Verification items for the finished model (mm, model axes). Face numbers are marked on the shaded views. Round coordinates to 2 decimals unless told otherwise and drop trailing zeros. Order: outer loops, then holes, each group sorted by start corner. A loop starts at its lowest first (then second) coordinate and runs counter-clockwise, first axis right, second up. Notation, with made-up numbers: (65.25, -16.5) -> (123.25, -16.5) arc R14 ccw to (123.25, -7.5) -> close; hole circle Ø2 at (4.5, -28.5). An arc over 180 degrees is marked (long way). Return JSON: item names as keys, results as strings. Group by question number.
Item 1: Sectioned sample at B-B on x = 0. Record the cut outline in (y, z).
Item 2: Depth check by flat-ended pin: pin 1 Ø2 at (y, z) = (17.5, 7.5) entering from -X; pin 2 Ø8 at (x, z) = (6.5, 18) entering from -Y; pin 3 Ø10 at (x, y) = (-31, 37.5) entering from +Z. Enter the tip coordinate at first touch or a pass-through.
Item 3: Sectioned sample at A-A on y = 0. Record the cut outline in (x, z), plus the area to 3 significant figures.
Item 4: Sectioned sample at D-D on z = 48. Record the cut outline in (x, y) (3 decimals), plus the area to 3 significant figures.
Item 5: Sectioned sample at C-C on z = 33. Give the number of separate pieces and of enclosed holes in the cut face, plus the area to 3 significant figures.
Item 6: Scan lines: probe 1 along Y at (x, z) = (0, 23.5); probe 2 along Y at (x, z) = (22.5, 36.5); probe 3 along X at (y, z) = (-5, 31). Record each from-to range of solid material in increasing order. Write a range as from..to.
Item 7: Draft check along X on the marked faces 1, 2 and 3. Enter one of: pulls with the +X half, pulls with the -X half, needs draft (parallel to the pull), parting line crosses it, or undercut.
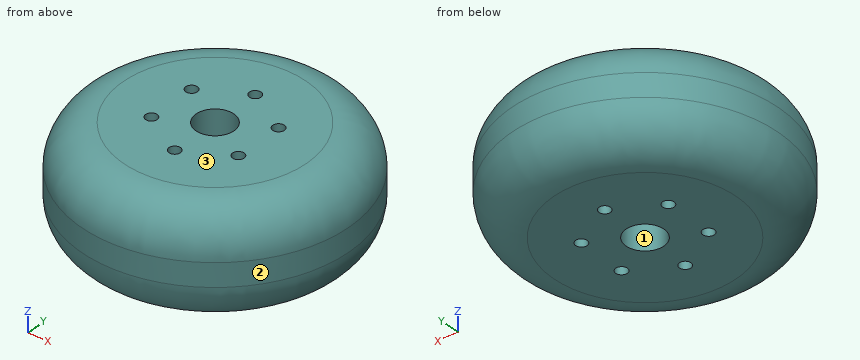
```python
from build123d import *

# Parameters (mm, degrees)
SKETCH1_R            = 63.5
SKETCH1_R_2          = 9
BOSS_EXTRUDE1_DEPTH  = 51
FILLET1_R            = 20
M5_CLEARANCE_HOLE1_D = 5.5


with BuildPart() as part:
    # Sketch1 → Boss-Extrude1 (new body)
    with BuildSketch(Plane.XY):
        Circle(SKETCH1_R)
        Circle(SKETCH1_R_2, mode=Mode.SUBTRACT)
    extrude(amount=BOSS_EXTRUDE1_DEPTH)

    # Fillet1
    fillet1_edges = [part.edges().sort_by_distance(p)[0] for p in [
        (-63.5, 0, 0),
        (-63.5, 0, 51),
    ]]
    fillet(fillet1_edges, radius=FILLET1_R)

    # M5 Clearance Hole1 (through all)
    with Locations(Plane.XY.offset(51)):
        with Locations((0, 23.75), (20.56810334, 11.875), (20.56810334, -11.875), (0, -23.75), (-20.56810334, -11.875), (-20.56810334, 11.875)):
            Hole(M5_CLEARANCE_HOLE1_D / 2)


solid = part.part
```
Recorded:
{
 "1": {"outline": "(-63.5, 20) arc R20 ccw to (-43.5, 0) -> (-26.5, 0) -> (-26.5, 51) -> (-43.5, 51) arc R20 ccw to (-63.5, 31) -> close; (-21, 0) -> (-9, 0) -> (-9, 51) -> (-21, 51) -> close; (9, 0) -> (21, 0) -> (21, 51) -> (9, 51) -> close; (26.5, 0) -> (43.5, 0) arc R20 ccw to (63.5, 20) -> (63.5, 31) arc R20 ccw to (43.5, 51) -> (26.5, 51) -> close"},
 "2": {"pin 1": "x = -57.31", "pin 2": "y = -63.43", "pin 3": "z = 51"},
 "3": {"outline": "(-63.5, 20) arc R20 ccw to (-43.5, 0) -> (-9, 0) -> (-9, 51) -> (-43.5, 51) arc R20 ccw to (-63.5, 31) -> close; (9, 0) -> (43.5, 0) arc R20 ccw to (63.5, 20) -> (63.5, 31) arc R20 ccw to (43.5, 51) -> (9, 51) -> close", "area": "5,220 mm²"},
 "4": {"outline": "circle Ø108.071 at (0, 0); hole circle Ø5.5 at (-20.568, -11.875); hole circle Ø5.5 at (-20.568, 11.875); hole circle Ø18 at (0, 0); hole circle Ø5.5 at (0, -23.75); hole circle Ø5.5 at (0, 23.75); hole circle Ø5.5 at (20.568, -11.875); hole circle Ø5.5 at (20.568, 11.875)", "area": "8,780 mm²"},
 "5": {"separate pieces": "1", "enclosed holes": "7", "area": "12,200 mm²"},
 "6": {"probe 1": "-63.5..-26.5, -21..-9, 9..21, 26.5..63.5", "probe 2": "-58.55..-13.83, -9.92..9.92, 13.83..58.55", "probe 3": "-63.3..-7.48, 7.48..63.3"},
 "7": {"face 1": "undercut", "face 2": "parting line crosses it", "face 3": "needs draft"}
}
